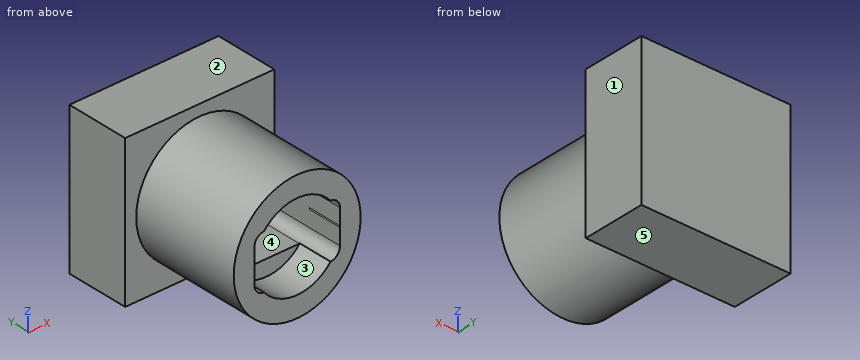
Autodesk Inventor part; units mm, degrees
ref_plane "YZ Plane" through (0, 0, 0) normal (1, 0, 0) x (0, 1, 0)
ref_plane "XZ Plane" through (0, 0, 0) normal (0, 1, 0) x (-1, 0, 0)
ref_plane "XY Plane" through (0, 0, 0) normal (0, 0, 1) x (1, 0, 0)
sketch "Sketch1" plane through (0, 0, 0) normal (0, 1, 0) x (-1, 0, 0)
  line L0 (14.5, -14.5) -> (-14.5, -14.5)
  line L1 (-14.5, -14.5) -> (-14.5, 14.5)
  line L2 (-14.5, 14.5) -> (14.5, 14.5)
  line L3 (14.5, 14.5) -> (14.5, -14.5)
  circle A0 centre (0, 0) radius 4
  dimension "d11" = 29
  dimension "d14" = 29
  dimension "d31" = 8
extrude "Extrusion1" add sketch "Sketch1" along normal blind 7 contours A0
sketch "Sketch2" plane through (0, 7, 0) normal (0, 1, 0) x (1, 0, 0)
  line L0 (-4.7, 4.7) -> (4.7, 4.7)
  line L1 (4.7, 4.7) -> (4.7, -4.7)
  line L2 (4.7, -4.7) -> (-4.7, -4.7)
  line L3 (-4.7, -4.7) -> (-4.7, 4.7)
  line L4 (14.5, 14.5) -> (-14.5, 14.5)
  line L5 (14.5, -14.5) -> (14.5, 14.5)
  line L6 (-14.5, -14.5) -> (14.5, -14.5)
  line L7 (-14.5, 14.5) -> (-14.5, -14.5)
  point P0 (0, 0)
  dimension "d15" = 9.8
  dimension "d16" = 9.8
  dimension "d17" = 9.8
  dimension "d18" = 9.8
  dimension "d32" = 9.4
  dimension "d50" = 29
extrude "Extrusion2" add sketch "Sketch2" along normal blind 4 contours L0 L1 L2 L3
sketch "Sketch3" plane through (0, 0, 0) normal (0, -1, 0) x (1, 0, 0)
  line L0 (-0.0005, -0.0003) -> (-0.0005, -1.7003)
  line L1 (-0.0005, -1.7003) -> (2.6995, -1.7003)
  line L2 (2.6995, -1.7003) -> (2.6995, 1.6997)
  line L3 (2.6995, 1.6997) -> (-2.7005, 1.6997)
  line L4 (-2.7005, 1.6997) -> (-2.7005, -1.7003)
  line L5 (-2.7005, -1.7003) -> (-0.0005, -1.7003)
  dimension "d42" = 1.7
  dimension "d43" = 2.7
  dimension "d44" = 3.4
  dimension "d45" = 5.4
extrude "Extrusion3" cut sketch "Sketch3" against normal blind 8.2
sketch "Sketch5" plane through (0, 0, 0) normal (0, -1, 0) x (1, 0, 0)
  circle A0 centre (0, 0) radius 2.7
  dimension "d35" = 5.4
extrude "Extrusion4" cut sketch "Sketch5" against normal blind 2.2
fillet "Fillet1" radius 0.635 4 edges at (2.6995, 4.1, 1.6997) (2.6995, 4.1, -1.7003) (-2.7005, 4.1, -1.7003) (-2.7005, 4.1, 1.6997)
equation "\"d14\" = d11"
equation "\"d16\" = d15"
equation "\"d17\" = d15"
equation "\"d18\" = d15"
equation "\"d42\" = 0.5 * d44"
properties part number "Motor_Key_Bearing_2_2"
Build history of the part. All positions in model axes, mm. Face numbers are marked on the shaded views. A direction names the side the tool comes from. Give positions to 0.01 mm unless a question says otherwise; leave off trailing zeros. Loops run counter-clockwise (first coordinate to the right, second up) from the corner with the lowest first, then second, coordinate; pieces in that order, holes last.
1) Band-saw the part on C-C on z = -2. List the corners of the cut face in (x, y), then the cut area to 3 significant figures.
Values follow:
outline: (-4.7, 7) - (-3.46, 7) - (-3.46, 0) - (-1.81, 0) - (-1.81, 2.2) - (1.81, 2.2) - (1.81, 0) - (3.46, 0) - (3.46, 7) - (4.7, 7) - (4.7, 11) - (-4.7, 11) - close
area: 78.1 mm2
2) 3-axis set-ups, long thin cutter, end or side, ignore diameter. For the marked faces 4 and 5: which of +Z, -Z, +X, -X, +Y, -Y reach the whole face in a straight line?
Values follow:
face 4: -Y
face 5: -Z, +X, -X, +Y, -Y
3) Two-plate mould, pull along Z, no slides. Class the marked faces 1, 2 and 3: released by +Z, released by -Z, zero draft, split by the parting line, or undercut.
Values follow:
face 1: zero draft
face 2: released by +Z
face 3: undercut
4) Band-saw the part on B-B on x = 0. List the corners of the cut face in (y, z), then the cut area to 3 significant figures.
Values follow:
outline: (0, -4) - (7, -4) - (7, -4.7) - (11, -4.7) - (11, 4.7) - (7, 4.7) - (7, 4) - (0, 4) - (0, 2.7) - (2.2, 2.7) - (2.2, 1.7) - (8.2, 1.7) - (8.2, -1.7) - (2.2, -1.7) - (2.2, -2.7) - (0, -2.7) - close
area: 61.3 mm2
5) Probe line 1 along Z through (x, y) = (0.25, 7.5); line 2 along Z through (x, y) = (-0.25, 5.5); line 3 along Y through (x, z) = (3.75, -1.5). List the from-to ranges inside material, lowest first.
Values follow:
line 1: z = -4.7 to -1.7, 1.7 to 4.7
line 2: z = -3.99 to -1.7, 1.7 to 3.99
line 3: y = 7 to 11
6) Band-saw the part on D-D on y = 2.75. List the corners of the cut face in (x, z) (1 decimal), then the cut area to 3 significant figures.
Values follow:
outline: circle Ø8 at (0, 0); hole (-2.7, -1.1) arc R0.6 ccw to (-2.1, -1.7) - (2.1, -1.7) arc R0.6 ccw to (2.7, -1.1) - (2.7, 1.1) arc R0.6 ccw to (2.1, 1.7) - (-2.1, 1.7) arc R0.6 ccw to (-2.7, 1.1) - close
area: 32.3 mm2
7) Drop flat-ended pins along their axis: P1, Ø2.5, axis at y = 5.5, z = -0.5, coming from the +X side; P2, Ø2, axis at x = -1, y = 5.5, coming from the +Z side; P3, Ø4, axis at x = 1.5, y = 1, coming from the -Z side. Give the stop position or say it passes through.
Values follow:
P1: stops at x = 4
P2: stops at z = 4
P3: stops at z = -4
8) Band-saw the part on A-A on y = 8. List the corners of the cut face in (x, z) (1 decimal).
Values follow:
outline: (-4.7, -4.7) - (4.7, -4.7) - (4.7, 4.7) - (-4.7, 4.7) - close; hole (-2.7, -1.1) arc R0.6 ccw to (-2.1, -1.7) - (2.1, -1.7) arc R0.6 ccw to (2.7, -1.1) - (2.7, 1.1) arc R0.6 ccw to (2.1, 1.7) - (-2.1, 1.7) arc R0.6 ccw to (-2.7, 1.1) - close
